Could you check a few things on this model? Use its own coordinates, in mm. Round coordinates to 2 decimals unless told otherwise and drop trailing zeros. Loops run counter-clockwise (first coordinate to the right, second up) from the corner with the lowest first, then second, coordinate; pieces in that order, holes last. Notation, with made-up numbers: (34, 66) - (58, 66) arc R24 ccw to (58, 91) - close; hole circle Ø5 at (16.25, 17). An arc over 180 degrees is marked (long way). Answer as CSV lines item,"result". Start each with the question number.
1) I'm going to push flat-ended pins straight in: pin 1 Ø10.5 at (x, z) = (0, -1.44) entering from +Y; pin 2 Ø1.5 at (y, z) = (-14, -26) entering from +X. Where does each tip first touch, or does it pass through?
2) Please list where these lines run through material, in increasing order: line 1 along Z through (x, y) = (-25.4, -6.25); line 2 along Z through (x, y) = (29, -15.75); line 3 along X through (y, z) = (-14.25, 22.5).
3) Suppose I cut it at C-C, the plane y = -12.5. Count the separate pieces of the cut face and the enclosed holes in it, then the cut area to 3 significant figures.
4) Suppose I cut it at B-B, the plane z = -5. Write out the boundary of the cut face in (x, y), then the cut area to 3 significant figures.
5) We'd pull the mould along Z, two halves only. Please class faces 1 (the face through (-32.31, -12.52, 18.66)), 2 (the face through (-56, -13, -44.495)), 3 (the face through (-27.29, -12.52, -35.34)), 4 (the face through (-1, -25.4, 11)): pulls with the +Z half, pulls with the -Z half, needs draft (parallel to the pull), parting line crosses it, or undercut.
6) Suppose I cut it at A-A, the plane x = -25.4. Write out the boundary of the cut face in (y, z).
```python
from build123d import *

# Parameters (mm, degrees)
F0_R     = 8.7067179479
F1_DEPTH = 25.4


with BuildPart() as f1:
    # F0 (on Front) → F1 (new body)
    with BuildSketch(Plane.XZ):
        with BuildLine():
            Line((57.1053996682, 29.9631231404), (57.1053996682, 44.4953776896))
            Line((57.1053996682, 44.4953776896), (31.7053996682, 44.4953776896))
            Line((31.7053996682, 44.4953776896), (31.7053996682, 29.9631231404))
            ThreePointArc((31.7053996682, 29.9631231404), (33.4841287064, 27.1922855677), (34.1067179479, 23.9590518177))
            ThreePointArc((34.1067179479, 23.9590518177), (33.4841287064, 20.7258180677), (31.7053996682, 17.9549804949))
            Line((31.7053996682, 17.9549804949), (31.7053996682, 4.5631231404))
            ThreePointArc((31.7053996682, 4.5631231404), (33.4841287064, 1.7922855677), (34.1067179479, -1.4409481823))
            ThreePointArc((34.1067179479, -1.4409481823), (33.4841287064, -4.6741819323), (31.7053996682, -7.4450195051))
            Line((31.7053996682, -7.4450195051), (31.7053996682, -20.8368768596))
            ThreePointArc((31.7053996682, -20.8368768596), (33.4841287064, -23.6077144323), (34.1067179479, -26.8409481823))
            ThreePointArc((34.1067179479, -26.8409481823), (33.4841287064, -30.0741819323), (31.7053996682, -32.8450195051))
            Line((31.7053996682, -32.8450195051), (31.7053996682, -44.4953776896))
            Line((31.7053996682, -44.4953776896), (46.8234342497, -44.4953776896))
            ThreePointArc((46.8234342497, -44.4953776896), (50.8, -43.5342302345), (54.7765657503, -44.4953776896))
            Line((54.7765657503, -44.4953776896), (57.1053996682, -44.4953776896))
            Line((57.1053996682, -44.4953776896), (57.1053996682, -32.8450195051))
            ThreePointArc((57.1053996682, -32.8450195051), (42.0932820521, -26.8409481823), (57.1053996682, -20.8368768596))
            Line((57.1053996682, -20.8368768596), (57.1053996682, -7.4450195051))
            ThreePointArc((57.1053996682, -7.4450195051), (42.0932820521, -1.4409481823), (57.1053996682, 4.5631231404))
            Line((57.1053996682, 4.5631231404), (57.1053996682, 17.9549804949))
            ThreePointArc((57.1053996682, 17.9549804949), (42.0932820521, 23.9590518177), (57.1053996682, 29.9631231404))
        make_face()
        with BuildLine():
            Line((31.7053996682, 29.9631231404), (31.7053996682, 44.4953776896))
            Line((31.7053996682, 44.4953776896), (6.3053996682, 44.4953776896))
            Line((6.3053996682, 44.4953776896), (6.3053996682, 29.9631231404))
            ThreePointArc((6.3053996682, 29.9631231404), (8.0841287064, 27.1922855677), (8.7067179479, 23.9590518177))
            ThreePointArc((8.7067179479, 23.9590518177), (8.0841287064, 20.7258180677), (6.3053996682, 17.9549804949))
            Line((6.3053996682, 17.9549804949), (6.3053996682, 4.5631231404))
            ThreePointArc((6.3053996682, 4.5631231404), (8.0841287064, 1.7922855677), (8.7067179479, -1.4409481823))
            ThreePointArc((8.7067179479, -1.4409481823), (8.0841287064, -4.6741819323), (6.3053996682, -7.4450195051))
            Line((6.3053996682, -7.4450195051), (6.3053996682, -20.8368768596))
            ThreePointArc((6.3053996682, -20.8368768596), (8.0841287064, -23.6077144323), (8.7067179479, -26.8409481823))
            ThreePointArc((8.7067179479, -26.8409481823), (8.0841287064, -30.0741819323), (6.3053996682, -32.8450195051))
            Line((6.3053996682, -32.8450195051), (6.3053996682, -44.4953776896))
            Line((6.3053996682, -44.4953776896), (21.4234342497, -44.4953776896))
            ThreePointArc((21.4234342497, -44.4953776896), (25.4, -43.5342302345), (29.3765657503, -44.4953776896))
            Line((29.3765657503, -44.4953776896), (31.7053996682, -44.4953776896))
            Line((31.7053996682, -44.4953776896), (31.7053996682, -32.8450195051))
            ThreePointArc((31.7053996682, -32.8450195051), (16.6932820521, -26.8409481823), (31.7053996682, -20.8368768596))
            Line((31.7053996682, -20.8368768596), (31.7053996682, -7.4450195051))
            ThreePointArc((31.7053996682, -7.4450195051), (16.6932820521, -1.4409481823), (31.7053996682, 4.5631231404))
            Line((31.7053996682, 4.5631231404), (31.7053996682, 17.9549804949))
            ThreePointArc((31.7053996682, 17.9549804949), (16.6932820521, 23.9590518177), (31.7053996682, 29.9631231404))
        make_face()
        with BuildLine():
            Line((6.3053996682, 29.9631231404), (6.3053996682, 44.4953776896))
            Line((6.3053996682, 44.4953776896), (-57.1053996682, 44.4953776896))
            Line((-57.1053996682, 44.4953776896), (-57.1053996682, 29.9631231404))
            ThreePointArc((-57.1053996682, 29.9631231404), (-47.56676625, 32.0431805241), (-42.0932820521, 23.9590518177))
            ThreePointArc((-42.0932820521, 23.9590518177), (-47.56676625, 15.8749231112), (-57.1053996682, 17.9549804949))
            Line((-57.1053996682, 17.9549804949), (-57.1053996682, 4.5631231404))
            ThreePointArc((-57.1053996682, 4.5631231404), (-47.56676625, 6.6431805241), (-42.0932820521, -1.4409481823))
            ThreePointArc((-42.0932820521, -1.4409481823), (-47.56676625, -9.5250768888), (-57.1053996682, -7.4450195051))
            Line((-57.1053996682, -7.4450195051), (-57.1053996682, -20.8368768596))
            ThreePointArc((-57.1053996682, -20.8368768596), (-47.56676625, -18.7568194759), (-42.0932820521, -26.8409481823))
            ThreePointArc((-42.0932820521, -26.8409481823), (-47.56676625, -34.9250768888), (-57.1053996682, -32.8450195051))
            Line((-57.1053996682, -32.8450195051), (-57.1053996682, -44.4953776896))
            Line((-57.1053996682, -44.4953776896), (-54.7765657503, -44.4953776896))
            ThreePointArc((-54.7765657503, -44.4953776896), (-50.8, -43.5342302345), (-46.8234342497, -44.4953776896))
            Line((-46.8234342497, -44.4953776896), (-29.3765657503, -44.4953776896))
            ThreePointArc((-29.3765657503, -44.4953776896), (-25.4, -43.5342302345), (-21.4234342497, -44.4953776896))
            Line((-21.4234342497, -44.4953776896), (-3.9765657503, -44.4953776896))
            ThreePointArc((-3.9765657503, -44.4953776896), (0, -43.5342302345), (3.9765657503, -44.4953776896))
            Line((3.9765657503, -44.4953776896), (6.3053996682, -44.4953776896))
            Line((6.3053996682, -44.4953776896), (6.3053996682, -32.8450195051))
            ThreePointArc((6.3053996682, -32.8450195051), (-8.7067179479, -26.8409481823), (6.3053996682, -20.8368768596))
            Line((6.3053996682, -20.8368768596), (6.3053996682, -7.4450195051))
            ThreePointArc((6.3053996682, -7.4450195051), (-8.7067179479, -1.4409481823), (6.3053996682, 4.5631231404))
            Line((6.3053996682, 4.5631231404), (6.3053996682, 17.9549804949))
            ThreePointArc((6.3053996682, 17.9549804949), (-8.7067179479, 23.9590518177), (6.3053996682, 29.9631231404))
        make_face()
        with Locations((-25.4, -26.8409481823)):
            Circle(F0_R, mode=Mode.SUBTRACT)
        with Locations((-25.4, -1.4409481823)):
            Circle(F0_R, mode=Mode.SUBTRACT)
        with Locations((-25.4, 23.9590518177)):
            Circle(F0_R, mode=Mode.SUBTRACT)
    extrude(amount=F1_DEPTH)


solid = f1.part
```
Filled sheet:
1,pin 1,"through"
1,pin 2,"x = 42.24"
2,line 1,"-43.53 to -35.55, -18.13 to -10.15, 7.27 to 15.25, 32.67 to 44.5"
2,line 2,"-44.31 to -34.77, -18.91 to -9.37, 6.49 to 16.03, 31.89 to 44.5"
2,line 3,"-42.22 to -33.98, -16.82 to -8.58, 8.58 to 16.82, 33.98 to 42.22"
3,separate pieces,"1"
3,enclosed holes,"9"
3,area,"6,680 mm²"
4,outline,"(-42.85, -25.4) - (-33.35, -25.4) - (-33.35, 0) - (-42.85, 0) - close; (-17.45, -25.4) - (-7.95, -25.4) - (-7.95, 0) - (-17.45, 0) - close; (7.95, -25.4) - (17.45, -25.4) - (17.45, 0) - (7.95, 0) - close; (33.35, -25.4) - (42.85, -25.4) - (42.85, 0) - (33.35, 0) - close"
4,area,"966 mm²"
5,face 1,"undercut"
5,face 2,"pulls with the -Z half"
5,face 3,"undercut"
5,face 4,"needs draft"
6,outline,"(-25.4, -43.53) - (0, -43.53) - (0, -35.55) - (-25.4, -35.55) - close; (-25.4, -18.13) - (0, -18.13) - (0, -10.15) - (-25.4, -10.15) - close; (-25.4, 7.27) - (0, 7.27) - (0, 15.25) - (-25.4, 15.25) - close; (-25.4, 32.67) - (0, 32.67) - (0, 44.5) - (-25.4, 44.5) - close"
